Model file for the job. Use its own axes, mm. A direction names the side the tool comes from. Round coordinates to 2 decimals unless told otherwise and drop trailing zeros. Loops run counter-clockwise (first coordinate to the right, second up) from the corner with the lowest first, then second, coordinate; pieces in that order, holes last. Notation, with made-up numbers: (85.25, -20.75) -> (94.25, -20.75) arc R18 cw to (94.25, 1.25) -> close; hole circle Ø2 at (69, -11.5). An arc over 180 degrees is marked (long way). Use a Markdown table: item, result.
from build123d import *

# Parameters (mm, degrees)
ESBO_O1_W                = 425
ESBO_O1_H                = 175
FLANGE_BASE1_DEPTH       = 4
ESBO_O11_W               = 10.6
ESBO_O11_H               = 90.6
CORTE_EXTRUS_O2_DEPTH    = 155
DOBRA_ESBO_ADA1_DEPTH    = 175
DOBRA_ESBO_ADA1_2_DEPTH  = 175
DOBRA_ESBO_ADA1_3_DEPTH  = 42.2
DOBRA_START              = 132.8
DOBRA_ESBO_ADA1_4_DEPTH  = 42.2
ESBO_O14_R               = 1.75
CORTE_EXTRUS_O3_DEPTH    = 6
ESBO_O15_W               = 10.6
ESBO_O15_H               = 91.1
CORTE_EXTRUS_O4_DEPTH    = 44
ESBO_O16_W               = 2
ESBO_O16_H               = 4
RESSALTO_EXTRUS_O1_DEPTH = 175


# Read off the part's stored shape, not the designer's step: Dobra esboçada1
# Sheet-metal steps are written as plain solids
with BuildPart() as part:
    # Esboço1 → Flange-base1 (new body)
    with BuildSketch(Plane.XY):
        with Locations((212.5, 87.5)):
            Rectangle(ESBO_O1_W, ESBO_O1_H)
    extrude(amount=-FLANGE_BASE1_DEPTH)

    # Esboço11 → Corte-extrusão2 (cut)
    with BuildSketch(Plane(origin=(0, 0, -4), x_dir=(-1, 0, 0), z_dir=(0, 0, -1))):
        Polygon((-425, 175), (-425, 0), (-410.6, 0), (-410.6, 42.2), (-410.6, 132.8), (-410.6, 175), align=None)
        with Locations((-405.3, 87.5)):
            Rectangle(ESBO_O11_W, ESBO_O11_H)
    extrude(amount=-CORTE_EXTRUS_O2_DEPTH, mode=Mode.SUBTRACT)

    # Dobra esboçada1 outline → Dobra esboçada1 (cut)
    with BuildSketch(Plane(origin=(0, 0, 0), x_dir=(1, 0, 0), z_dir=(0, 1, 0))):
        with BuildLine():
            ThreePointArc((193.564342649, 4), (203.956647495, 2.990565198), (213.960420704, 0))
            Line((213.960420704, 0), (410.6, 0))
            Line((410.6, 0), (410.6, 4))
            Line((410.6, 4), (193.564342649, 4))
        make_face()
    extrude(amount=DOBRA_ESBO_ADA1_DEPTH, mode=Mode.SUBTRACT)

    # Dobra esbo_ada1 2 outline → Dobra esbo_ada1 2 (add)
    with BuildSketch(Plane(origin=(0, 0, 0), x_dir=(1, 0, 0), z_dir=(0, 1, 0))):
        with BuildLine():
            Line((277.537342774, -170.206337672), (281.401046079, -169.171061491))
            Line((281.401046079, -169.171061491), (245.724337269, -36.023771564))
            ThreePointArc((245.724337269, -36.023771564), (234.067724606, -14.286192444), (213.960420704, 0))
            Line((213.960420704, 0), (193.564342649, 0))
            ThreePointArc((193.564342649, 0), (224.0024141, -10.332332985), (241.860633964, -37.059047745))
            Line((241.860633964, -37.059047745), (277.537342774, -170.206337672))
        make_face()
    extrude(amount=DOBRA_ESBO_ADA1_2_DEPTH)

    # Dobra esbo_ada1 3 outline → Dobra esbo_ada1 3 (add)
    with BuildSketch(Plane(origin=(0, 0, 0), x_dir=(1, 0, 0), z_dir=(0, 1, 0))):
        Polygon((280.280824652, -180.44515143), (284.144527957, -179.40987525), (281.401046079, -169.171061491), (277.537342774, -170.206337672), align=None)
    extrude(amount=DOBRA_ESBO_ADA1_3_DEPTH)

    # Dobra esbo_ada1 4 outline → Dobra esbo_ada1 4 (add)
    with BuildSketch(Plane(origin=(0, 0, 0), x_dir=(1, 0, 0), z_dir=(0, 1, 0)).offset(DOBRA_START)):
        Polygon((280.280824652, -180.44515143), (284.144527957, -179.40987525), (281.401046079, -169.171061491), (277.537342774, -170.206337672), align=None)
    extrude(amount=DOBRA_ESBO_ADA1_4_DEPTH)

    # Esboço14 → Corte-extrusão3 (cut)
    with BuildSketch(Plane(origin=(220.257984945, 0, -59.017949192), x_dir=(-0.25881904510251796, 0, -0.9659258262890691), z_dir=(0.9659258262890691, 0, -0.25881904510251796))):
        with Locations((-241.688647392, 13.1)):
            Circle(ESBO_O14_R)
        with Locations((-241.688647392, 23.6)):
            Circle(ESBO_O14_R)
    corte_extrus_o3 = extrude(amount=-CORTE_EXTRUS_O3_DEPTH, mode=Mode.SUBTRACT)

    # Espelhar1: Corte-extrusão3 across plane
    add(corte_extrus_o3.mirror(Plane(origin=(0, 87.5, 0), x_dir=(0, 0, 1), z_dir=(0, -1, 0))), mode=Mode.SUBTRACT)

    # Esboço15 → Corte-extrusão4 (cut)
    with BuildSketch(Plane(origin=(220.257984945, 0, -59.017949192), x_dir=(-0.25881904510251796, 0, -0.9659258262890691), z_dir=(0.9659258262890691, 0, -0.25881904510251796))):
        with Locations((-241.538647392, 87.5)):
            Rectangle(ESBO_O15_W, ESBO_O15_H)
    extrude(amount=-CORTE_EXTRUS_O4_DEPTH, mode=Mode.SUBTRACT)

    # Esboço16 → Ressalto-extrusão1 (add)
    with BuildSketch(Plane.XZ):
        with Locations((-1, -2)):
            Rectangle(ESBO_O16_W, ESBO_O16_H)
    extrude(amount=-RESSALTO_EXTRUS_O1_DEPTH)


solid = part.part
Q1. Band-saw the part on C-C, the plane y = 67. Give the cut face in (x, z).
Results list:
| item | result |
|---|---|
| outline | (-2, -4) -> (193.56, -4) arc R54 ccw to (245.72, 36.02) -> (281.4, 169.17) -> (277.54, 170.21) -> (241.86, 37.06) arc R50 cw to (193.56, 0) -> (-2, 0) -> close |
Q2. Flat gauge pins, fed straight in: pin 1 (5 mm diameter, centred on y = 83, z = 30.5, fed in from +X); pin 2 (3.5 mm diameter, centred on x = 281, z = 173, fed in from -Y); pin 3 (1 mm diameter, centred on y = 50.5, z = 114, fed in from -X); pin 4 (5 mm diameter, centred on x = 186, y = 80, fed in from +Z). Where does each tip first touch, or does it go through?
Results list:
| item | result |
|---|---|
| pin 1 | stops at x = 244.82 |
| pin 2 | stops at y = 0 |
| pin 3 | stops at x = 262.34 |
| pin 4 | stops at z = 0 |
Q3. Band-saw the part on D-D, the plane z = 160.5. Give the cut face in (x, y).
Results list:
| item | result |
|---|---|
| outline | (274.94, 0) -> (279.08, 0) -> (279.08, 175) -> (274.94, 175) -> close |
Q4. Band-saw the part on B-B, the plane x = 30.5. Give the cut face in (y, z).
Results list:
| item | result |
|---|---|
| outline | (0, -4) -> (175, -4) -> (175, 0) -> (0, 0) -> close |
Q5. Tool access for faces 1 (the face through (94, 86, -4)), 2 (the face through (94, 86, 0)): list every direction of +Z, -Z, +X, -X, +Y, -Y with a clear straight run to the whole face (end or side of a thin tool).
Results list:
| item | result |
|---|---|
| face 1 | -Z, +X, -X, +Y, -Y |
| face 2 | +Z, -X, +Y, -Y |
Q6. Band-saw the part on A-A, the plane y = 33. Give the cut face in (x, z), plus the area to 3 significant figures.
Results list:
| item | result |
|---|---|
| outline | (-2, -4) -> (193.56, -4) arc R54 ccw to (245.72, 36.02) -> (284.14, 179.41) -> (280.28, 180.45) -> (241.86, 37.06) arc R50 cw to (193.56, 0) -> (-2, 0) -> close |
| area | 1,650 mm² |
Q7. Drill centre lines: L1, parallel to Z at x = 107.5, y = 48; L2, parallel to X at y = 165.5, z = 99; L3, parallel to X at y = 65, z = 72. Where is each one in solid material? Low to high. Write a range as from..to.
Results list:
| item | result |
|---|---|
| L1 | z = -4..0 |
| L2 | x = 258.46..262.6 |
| L3 | x = 251.22..255.36 |
